Design review of the part shown in the three views and the two pictorial views. Dimensions are in mm from the part's minimum x, y and z. A direction names the side the tool comes from. Round coordinates to 2 decimals unless told otherwise and drop trailing zeros. Loops run counter-clockwise (first coordinate to the right, second up) from the corner with the lowest first, then second, coordinate; pieces in that order, holes last. Notation, with made-up numbers: (76.5, 2.5) - (80.5, 2.5) arc R27 ccw to (80.5, 39.5) - close; hole circle Ø7 at (54.5, 3). An arc over 180 degrees is marked (long way). Return JSON: item names as keys, results as strings. Group by question number.
(1) Wall thickness on L1, parallel to Z at x = 5.25, y = 9.25; L2, parallel to X at y = 10, z = 5; L3, parallel to Y at x = 3.25, z = 7: over which ranges is each line inside the solid? List them lowest first. Write a range as [from, to].
(2) We need section C-C, the plane x = 5.25. Write out the cut boundary in (y, z), and give its area (3 significant figures).
(3) For the marked faces 1, 2 and 3, list the 3-axis set-ups (+Z, -Z, +X, -X, +Y, -Y) from which the entire face can be reached by the end or side of a thin tool; tool diameter is ignored.
(4) We need section B-B, the plane z = 1.5. Write out the cut boundary in (x, y), and give its area (3 significant figures).
(5) We need section D-D, the plane y = 2.5. Write out the cut boundary in (x, z), and give its area (3 significant figures).
(6) Clearance check with flat-ended pins moving along their axes: pin 1 (4 mm diameter, centred on x = 1.5, y = 4, fed in from +Z); pin 2 (1.6 mm diameter, centred on x = 0.5, z = 1, fed in from +Y); pin 3 (0.6 mm diameter, centred on y = 1, z = 7, fed in from -X); pin 4 (2 mm diameter, centred on x = 5.5, y = 6.5, fed in from +Z). State where each tip first meets the part, or that it passes through.
(7) We need section A-A, the plane y = 4. Write out the cut boundary in (x, z), and give its area (3 significant figures).
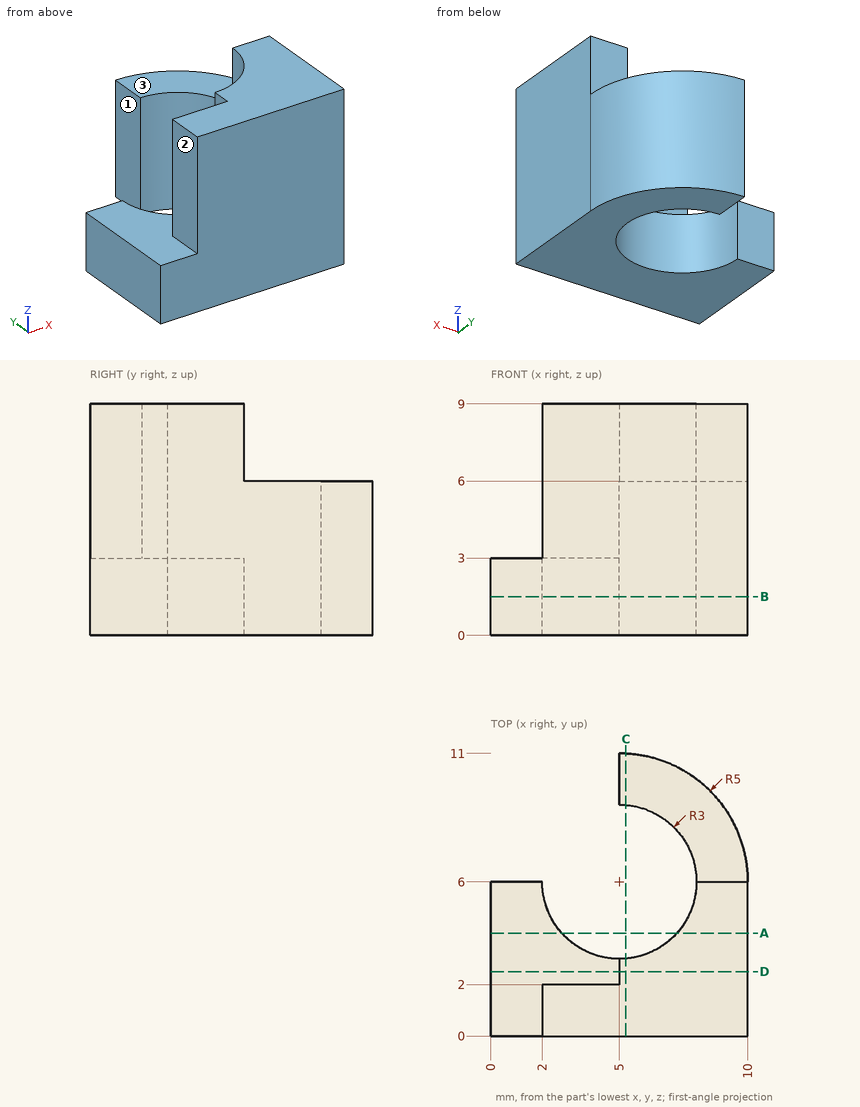
Solutions:
{
 "1": {"L1": "[0, 6]", "L2": "[5, 8]", "L3": "[0, 2]"},
 "2": {"outline": "(0, 0) - (3.01, 0) - (3.01, 9) - (0, 9) - close; (8.99, 0) - (10.99, 0) - (10.99, 6) - (8.99, 6) - close", "area": "39.1 mm^2"},
 "3": {"face 1": "+Z, -Z, -X, +Y", "face 2": "+Z, -X, +Y, -Y", "face 3": "+Z, +X, -X, +Y"},
 "4": {"outline": "(0, 0) - (10, 0) - (10, 6) arc R5 ccw to (5, 11) - (5, 9) arc R3 cw (long way) to (2, 6) - (0, 6) - close", "area": "58.4 mm^2"},
 "5": {"outline": "(0, 0) - (10, 0) - (10, 9) - (5, 9) - (5, 3) - (0, 3) - close", "area": "60.0 mm^2"},
 "6": {"pin 1": "z = 3", "pin 2": "y = 6", "pin 3": "x = 2", "pin 4": "through"},
 "7": {"outline": "(0, 0) - (2.76, 0) - (2.76, 3) - (0, 3) - close; (7.24, 0) - (10, 0) - (10, 9) - (7.24, 9) - close", "area": "33.2 mm^2"}
}
